Autodesk Inventor part; units mm, degrees
ref_plane "YZ Plane" through (0, 0, 0) normal (1, 0, 0) x (0, 1, 0)
ref_plane "XZ Plane" through (0, 0, 0) normal (0, 1, 0) x (-1, 0, 0)
ref_plane "XY Plane" through (0, 0, 0) normal (0, 0, 1) x (1, 0, 0)
sketch "Sketch1" plane through (0, 0, 0) normal (0, 1, 0) x (-1, 0, 0)
  line L0 (0, 0) -> (0, -34.9)
  line L1 (0, 0) -> (-4, 0) construction
  line L2 (0, -34.9) -> (-4, -34.9) construction
  line L3 (0, 0) -> (-5, 0)
  arc A0 (5, 0) -> (-5, 0) centre (0, 0) ccw
  line L4 (-5, 0) -> (-5, -34.9)
  arc A1 (-5, -34.9) -> (5, -34.9) centre (0, -34.9) ccw
  line L5 (5, -34.9) -> (5, 0)
  dimension "d11" = 34.9
  dimension "d12" = 5
  dimension "d13" = 90
  dimension "d14" = 34.9
extrude "Extrusion1" add sketch "Sketch1" along normal blind 5.5
sketch "Sketch2" plane through (0, 5.5, 0) normal (0, 1, 0) x (1, 0, 0)
  circle A0 centre (0, 0) radius 2.655
  line L0 (0, 0) -> (0, 34.9)
  circle A1 centre (0, 34.9) radius 2.655
  dimension "d7" = 5.31
  dimension "d8" = 34.9
  dimension "d9" = 5.31
sketch "Sketch3" plane through (0, 0, 0) normal (0, -1, 0) x (1, 0, 0)
  circle A0 centre (0, 0) radius 1.9
  line L0 (0, 0) -> (0, -34.9)
  circle A1 centre (0, -34.9) radius 1.9
  dimension "d15" = 3.8
  dimension "d16" = 34.9
  dimension "d17" = 3.8
extrude "Extrusion2" cut sketch "Sketch3" against normal blind 1.2
sketch "Sketch4" plane through (0, 1.2, -34.9) normal (0, -1, 0) x (1, 0, 0)
  circle A0 centre (0, 0) radius 1.9
  circle A1 centre (0, 0) radius 1.9
  circle A2 centre (0, 34.9) radius 1.9
sketch "Sketch5" plane through (5, 0, 0) normal (1, 0, 0) x (0, 0, -1)
  line L0 (0, 0) -> (0, 5.5)
  line L1 (0, 0) -> (0, 5.5)
hole "Hole1" at (0, 5.5, 0) at (0, 5.5, -34.9) direction (0, -1, 0) diameter 5.1 depth 4 tip angle 118 countersink diameter 5.31 countersink angle 3.01
thicken "Thicken1" operation add thickness 2 both sides no extend neighbours yes toward (-0.9967573, 0, -0.0804666) faces at (-4.9838, 1.8333, -35.3023) (5, 1.8333, -23.2667) (-5, 1.8333, -11.6333) (-4.9838, 3.6667, 0.4023)
properties part number "Rod_constraint"
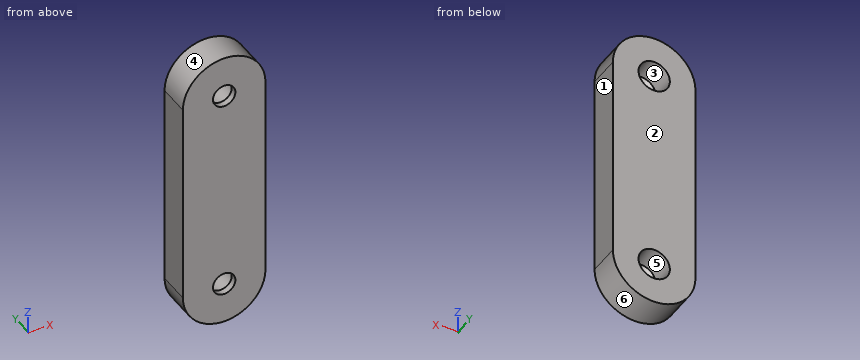
CAD build for the part. Positions are in the model's coordinates, mm. Face numbers are marked on the shaded views. A direction names the side the tool comes from. Round coordinates to 2 decimals unless told otherwise and drop trailing zeros. Order: outer loops, then holes, each group sorted by start corner. A loop starts at its lowest first (then second) coordinate and runs counter-clockwise, first axis right, second up. Notation, with made-up numbers: (-28, 69.5) - (8, 69.5) arc R14 cw to (8, 86.5) - close; hole circle Ø5 at (48.25, 71.5). An arc over 180 degrees is marked (long way). Use CSV: the item, a comma, the result in double quotes. Start each with the question number.
1) Saw through at A-A (y = 3.8). List the corners of the cut face in (x, z).
2) Tool access for the marked faces 5 and 6: list every direction of +Z, -Z, +X, -X, +Y, -Y with a clear straight run to the whole face (end or side of a thin tool).
3) Pin check, flat tips, straight feed: pin 1 Ø3 at (x, z) = (0, -34.9) entering from -Y; pin 2 Ø2 at (x, y) = (2.5, 4) entering from +Z. Stop position of each tip, or through.
4) Saw through at C-C (z = -38). List the corners of the cut face in (x, y), and give its area (3 significant figures).
5) Saw through at D-D (y = 0.65). List the corners of the cut face in (x, z), and give its area (3 significant figures).
6) Wall check: L1, parallel to Z at x = 0, y = 0.85; L2, parallel to Z at x = 0, y = 1.55; L3, parallel to X at y = 0.45, z = -34.9. Give the ranges that are in metal, low to high. Write a range as [from, to].
7) Saw through at B-B (x = -1). Count the separate pieces of the cut face and the enclosed holes in it, and give its area (3 significant figures).
8) Two-plate mould, pull along X, no slides. Class the marked faces 1, 2, 3 and 4: pulls with the +X half, pulls with the -X half, needs draft (parallel to the pull), parting line crosses it, or undercut.
Values follow:
1,outline,"(-7, -34.9) arc R7 ccw to (7, -34.9) - (7, 0) arc R7 ccw to (-7, 0) - close; hole circle Ø5.22 at (0, -34.9); hole circle Ø5.22 at (0, 0)"
2,face 5,"+Y"
2,face 6,"-Z, +Y, -Y"
3,pin 1,"passes through"
3,pin 2,"stops at z = 6.84"
4,outline,"(-6.28, 0) - (6.28, 0) - (6.28, 5.5) - (-6.28, 5.5) - close"
4,area,"69.0 mm2"
5,outline,"(-7, -34.9) arc R7 ccw to (7, -34.9) - (7, 0) arc R7 ccw to (-7, 0) - close; hole circle Ø3.8 at (0, -34.9); hole circle Ø3.8 at (0, 0)"
5,area,"620 mm2"
6,L1,"z = [-41.9, -36.8], [-33, -1.9], [1.9, 7]"
6,L2,"z = [-41.9, -37.45], [-32.35, -2.55], [2.55, 7]"
6,L3,"x = [-7, -1.9], [1.9, 7]"
7,separate pieces,"3"
7,enclosed holes,"0"
7,area,"219 mm2"
8,face 1,"pulls with the +X half"
8,face 2,"needs draft"
8,face 3,"undercut"
8,face 4,"parting line crosses it"
